The figure shows three views and two pictorial views of one solid part (mm, origin at its lowest corner). Answer the questions. Coordinates: 2 decimals unless noted, no trailing zeros. Order: outer loops, then holes, each group sorted by start corner. A loop starts at its lowest first (then second) coordinate and runs counter-clockwise, first axis right, second up. Notation, with made-up numbers: (84, -32) - (140, -32) arc R28 ccw to (140, -1) - close; hole circle Ø2 at (75, -38.75). An arc over 180 degrees is marked (long way). Use one line per item in the form item = value. Start each with the question number.
Item 1: Consider line 1 along Z through (x, y) = (9, 3.25) (1 decimal); line 2 along Z through (x, y) = (10.25, 1.75) (1 decimal); line 3 along Y through (x, z) = (5.5, 2.5). Determine where each line is inside the solid, lowest interval first. Write a range as [from, to].
Item 2: Section B-B, the plane x = 2.5 is taken. Write down the section's boundary in (y, z) (1 decimal).
Item 3: This flat-tipped pin is pushed along its axis until it touches: pin 1 Ø1.5 at (x, z) = (2.5, 1) entering from -Y. Where does it stop, or does it pass through?
Item 4: Section A-A, the plane x = 16.75 is taken. Write down the section's boundary in (y, z).
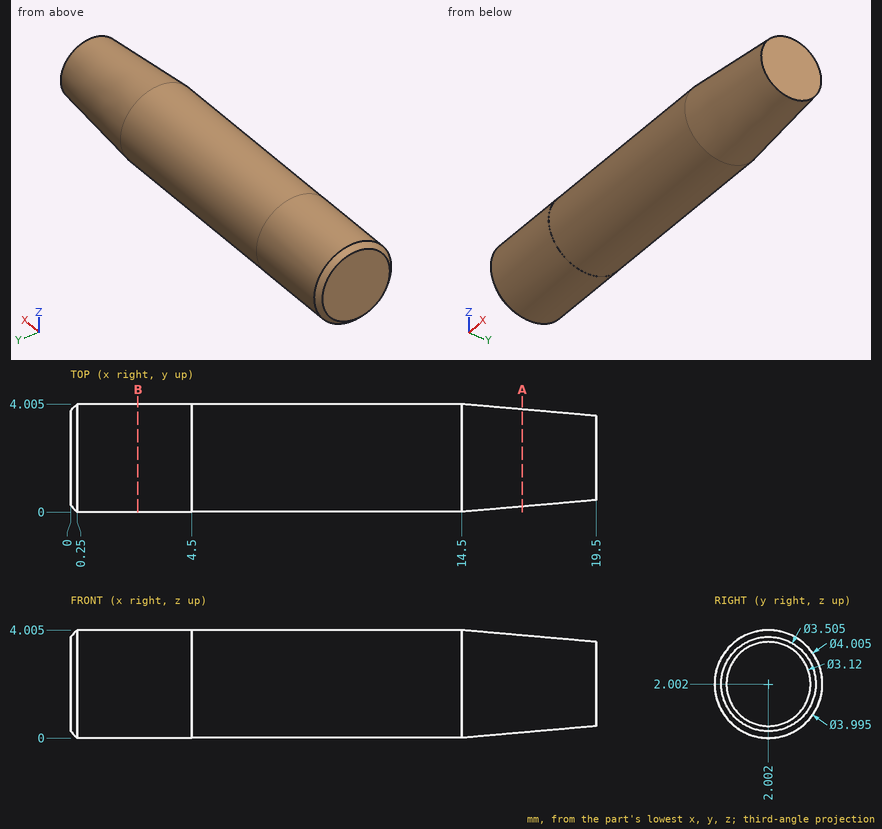
Response:
q1.line_1 = [0.4, 3.6]
q1.line_2 = [0, 4]
q1.line_3 = [0.07, 3.94]
q2.outline = circle Ø4 at (2, 2)
q3.pin_1 = 0.02
q4.outline = circle Ø3.6 at (2, 2)
